```python
from build123d import *

# Parameters (mm, degrees)
F0_R      = 20
F1_DEPTH  = 97
F2_T      = -6
F3_R      = 2
F4_DEPTH  = 40
F5_R      = 3
F6_R      = 5
F7_DEPTH  = 20.001
F8_R      = 5
F9_DEPTH  = 20.001
F10_R     = 5
F11_DEPTH = 194.001


with BuildPart() as f1:
    # F0 (on Right) → F1 (new body, symmetric)
    with BuildSketch(Plane.YZ):
        Circle(F0_R)
    extrude(amount=F1_DEPTH, both=True)

    # F2
    f2_openings = [f1.faces().sort_by_distance(p)[0] for p in [
        (97, 0, 0),
    ]]
    offset(amount=F2_T, openings=f2_openings)

    # F3 (on face) → F4 (cut)
    with BuildSketch(Plane.YZ.offset(97)):
        with Locations((17, 0)):
            Circle(F3_R)
        with Locations((12.020815, -12.020815)):
            Circle(F3_R)
        with Locations((-12.020815, -12.020815)):
            Circle(F3_R)
        with Locations((-17, 0)):
            Circle(F3_R)
        with Locations((12.020815, 12.020815)):
            Circle(F3_R)
        with Locations((-12.020815, 12.020815)):
            Circle(F3_R)
    extrude(amount=-F4_DEPTH, mode=Mode.SUBTRACT)

    # F5
    f5_edges = [f1.edges().sort_by_distance(p)[0] for p in [
        (-97, -20, 0),
    ]]
    fillet(f5_edges, radius=F5_R)

    # F6 (on Top) → F7 (cut, through all)
    with BuildSketch(Plane.XY):
        with Locations((-41, 0)):
            Circle(F6_R)
        with Locations((47, 0)):
            Circle(F6_R)
    extrude(amount=-F7_DEPTH, mode=Mode.SUBTRACT)

    # F8 (on Top) → F9 (cut, through all)
    with BuildSketch(Plane.XY):
        with Locations((3, 0)):
            Circle(F8_R)
    extrude(amount=F9_DEPTH, mode=Mode.SUBTRACT)

    # F10 (on face) → F11 (cut, through all)
    with BuildSketch(Plane(origin=(-97, 0, 0), x_dir=(0, -1, 0), z_dir=(-1, 0, 0))):
        with Locations((0, 9)):
            Circle(F10_R)
    extrude(amount=-F11_DEPTH, mode=Mode.SUBTRACT)


solid = f1.part
```
Geometry: final body of the model. Coordinates: model frame, mm. A direction names the side the tool comes from. Coordinates: 2 decimals unless noted, no trailing zeros. Order: outer loops, then holes, each group sorted by start corner. A loop starts at its lowest first (then second) coordinate and runs counter-clockwise, first axis right, second up. Notation, with made-up numbers: (45, -27.5) -> (64, -27.5) arc R25 cw to (64, -14.5) -> close; hole circle Ø3 at (76, -6). An arc over 180 degrees is marked (long way). Write item = value, one per line.
(1) Pin query (flat end, axial travel): pin 1 Ø5 at (x, y) = (-13.5, 15) entering from +Z; pin 2 Ø1.5 at (x, z) = (19, 11.5) entering from -Y; pin 3 Ø14 at (y, z) = (0.5, 6.5) entering from +X. Return the tip coordinate at first contact, or that it passes through.
Solved:
pin_1 = 15.61
pin_2 = -16.87
pin_3 = -91
(2) Access query for faces 4 (the cylindrical face through (42, 0, -16)), 5 (the flat face through (97, -8, 12)), 6 (the flat face through (57, 17, 0)). Directions: +Z, -Z, +X, -X, +Y, -Y. A direction counts if a zero-diameter tool reaches every point of the face in a straight line with its end or side. Return the directions, or none.
Solved:
face_4 = -Z
face_5 = +Z, -Z, +X, +Y, -Y
face_6 = +X
(3) Line query: line 1 (X direction, y = 0, z = -14.5); line 2 (Z direction, x = -29, y = 1); line 3 (X direction, y = 0, z = 16). Output: solid intervals per line, ascending.
Solved:
line_1 = -97 to -46, -36 to 42, 52 to 97
line_2 = -19.97 to -13.96, 13.96 to 19.97
line_3 = -97 to -2, 8 to 97
(4) Pull-direction query (Z, two-part tool) for faces 1 (the flat face through (57, -17, 0)), 2 (the cylindrical face through (2.837, 10.752, 16.864)), 3 (the cylindrical face through (5.307, -4.436, 16.49)); classes: pulls with the +Z half, pulls with the -Z half, needs draft (parallel to the pull), parting line crosses it, or undercut.
Solved:
face_1 = undercut
face_2 = parting line crosses it
face_3 = needs draft
(5) Cut plane B-B on x = 19.5. Return loops of the section in (y, z), plus the area to 3 significant figures.
Solved:
outline = circle Ø40 at (0, 0); hole circle Ø28 at (0, 0)
area = 641 mm²
(6) Cut plane A-A on x = 65. Return loops of the section in (y, z).
Solved:
outline = circle Ø40 at (0, 0); hole circle Ø4 at (-17, 0); hole circle Ø4 at (-12.02, -12.02); hole circle Ø4 at (-12.02, 12.02); hole circle Ø28 at (0, 0); hole circle Ø4 at (12.02, -12.02); hole circle Ø4 at (12.02, 12.02); hole circle Ø4 at (17, 0)
